Input: dimensioned drawing with shaded views. Units: mm. Origin: part minimum x, y, z. Coordinates: 2 decimals unless noted, no trailing zeros. Loops run counter-clockwise (first coordinate to the right, second up) from the corner with the lowest first, then second, coordinate; pieces in that order, holes last. Notation, with made-up numbers: (58.25, 70) - (73.25, 70) arc R7 cw to (73.25, 80) - close; hole circle Ø6 at (55.5, 88). An arc over 180 degrees is marked (long way). Use one line per item in the form item = value. Start each with the question number.
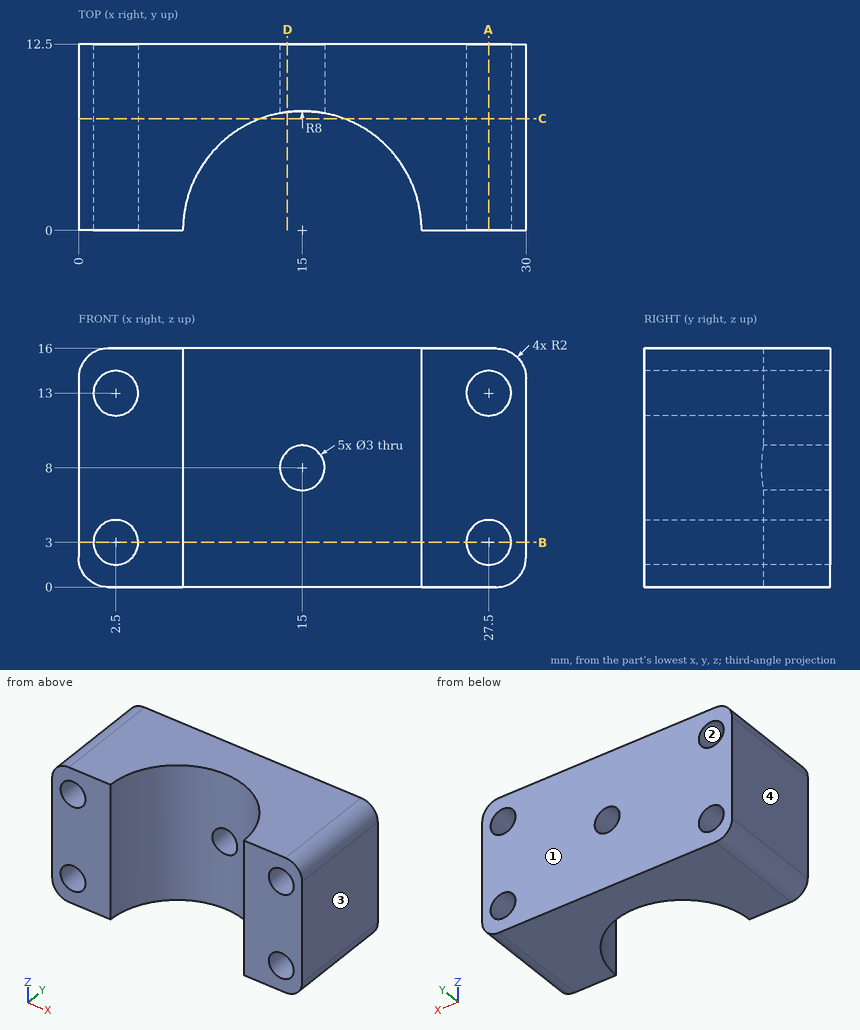
(1) Cut plane A-A, the plane x = 27.5. Output: boundary loops of the cut face in (y, z).
(2) Cut plane B-B, the plane z = 3. Output: boundary loops of the cut face in (x, y), plus the area to 3 significant figures.
(3) Material intervals for line 1 (Z direction, x = 2.5, y = 3.5); line 2 (X direction, y = 8.75, z = 3); line 3 (X direction, y = 9.2, z = 8), sorted ascending.
(4) Cut plane D-D, the plane x = 14. Output: boundary loops of the cut face in (y, z).
(5) Mould query, pull axis X, two halves, no side actions, for the marked faces 1, 2, 3 and 4. Classes: +X half, -X half, draft (parallel to the pull), parting line (faces both ways), or undercut.
(6) Contact query for flat-ended pins moving along their axis: pin 1 (4 mm diameter, centred on y = 9, z = 2, fed in from -X); pin 2 (2.5 mm diameter, centred on x = 15, z = 8, fed in from +Y). Output: stop coordinate, or through.
(7) Cut plane C-C, the plane y = 7.5. Output: boundary loops of the cut face in (x, z).
Recorded:
q1.outline = (0, 0) - (12.5, 0) - (12.5, 1.5) - (0, 1.5) - close; (0, 4.5) - (12.5, 4.5) - (12.5, 11.5) - (0, 11.5) - close; (0, 14.5) - (12.5, 14.5) - (12.5, 16) - (0, 16) - close
q2.outline = (0, 0) - (1, 0) - (1, 12.5) - (0, 12.5) - close; (4, 0) - (7, 0) arc R8 cw to (23, 0) - (26, 0) - (26, 12.5) - (4, 12.5) - close; (29, 0) - (30, 0) - (30, 12.5) - (29, 12.5) - close
q2.area = 199 mm²
q3.line_1 = 0 to 1.5, 4.5 to 11.5, 14.5 to 16
q3.line_2 = 0 to 1, 4 to 26, 29 to 30
q3.line_3 = 0 to 13.5, 16.5 to 30
q4.outline = (7.94, 0) - (12.5, 0) - (12.5, 6.88) - (7.94, 6.88) - close; (7.94, 9.12) - (12.5, 9.12) - (12.5, 16) - (7.94, 16) - close
q5.face_1 = draft
q5.face_2 = undercut
q5.face_3 = +X half
q5.face_4 = -X half
q6.pin_1 = 0
q6.pin_2 = through
q7.outline = (0, 2) arc R2 ccw to (2, 0) - (12.22, 0) - (12.22, 16) - (2, 16) arc R2 ccw to (0, 14) - close; (17.78, 0) - (28, 0) arc R2 ccw to (30, 2) - (30, 14) arc R2 ccw to (28, 16) - (17.78, 16) - close; hole circle Ø3 at (2.5, 3); hole circle Ø3 at (2.5, 13); hole circle Ø3 at (27.5, 3); hole circle Ø3 at (27.5, 13)
